from build123d import *

# Parameters (mm, degrees)
F0_W     = 45.72
F0_H     = 3.47472
F1_DEPTH = 3.47472
F3_DEPTH = 3.47472
F5_DEPTH = 38.1
F6_W     = 45.72
F6_H     = 0.254
F7_DEPTH = 0.508
F8_R     = 0.50799


# Not quite as in the source:
# - a fillet or chamfer is up to 0.001 mm smaller than in the source, because OpenCascade refuses the exact size


with BuildPart() as f1:
    # F0 (on Front) → F1 (new body)
    with BuildSketch(Plane.XZ):
        with Locations((0, -4.3103059118)):
            Rectangle(F0_W, F0_H)
    extrude(amount=F1_DEPTH)

    # F2 (on face) → F3 (join)
    with BuildSketch(Plane.XZ.offset(3.47472)):
        Polygon((-13.929602997, -2.5729459118), (-17.4304175377, -2.5729459118), (-24.6292689013, -61.2028853004), (-21.1804489373, -61.6263471453), align=None)
        Polygon((21.1804489373, -61.6263471453), (24.6292689013, -61.2028853004), (17.4304175377, -2.5729459118), (13.929602997, -2.5729459118), align=None)
    extrude(amount=-F3_DEPTH)

    # F4 (on Right) → F5 (cut, symmetric)
    with BuildSketch(Plane.YZ):
        Polygon((-3.47472, -2.9995878813), (0, -2.5729459118), (-3.47472, -2.5729459118), align=None)
        Polygon((0, -60.7762433309), (-3.47472, -61.2028853004), (-3.47472, -61.962287873), (0, -61.962287873), align=None)
    extrude(amount=F5_DEPTH, both=True, mode=Mode.SUBTRACT)

    # F6 (on face) → F7 (cut)
    with BuildSketch(Plane.XZ.offset(3.47472)):
        with Locations((0, -6.1746659118)):
            Rectangle(F6_W, F6_H)
    extrude(amount=-F7_DEPTH, mode=Mode.SUBTRACT)

    # F8 (radius 0.508 in the source; OpenCascade refuses exactly that, so slightly less here)
    f8_edges = [f1.edges().sort_by_distance(p)[0] for p in [
        (0, -3.47472, -2.999588),
        (22.86, 0, -4.310306),
        (22.86, -1.73736, -6.047666),
        (22.86, -3.47472, -4.523627),
        (22.86, -1.73736, -2.786267),
        (21.258758, -3.47472, -33.752276),
        (-17.757943, -3.47472, -33.752276),
        (-21.258758, -3.47472, -33.752276),
        (-22.86, 0, -4.310306),
        (-22.86, -1.73736, -2.786267),
        (-22.86, -3.47472, -4.523627),
        (-22.86, -1.73736, -6.047666),
        (17.757943, -3.47472, -33.752276),
        (20.35853, 0, -6.047666),
        (17.716157, 0, -33.411955),
        (0, 0, -6.047666),
        (-20.35853, 0, -6.047666),
        (-21.216972, 0, -33.411955),
        (-17.716157, 0, -33.411955),
        (21.216972, 0, -33.411955),
        (0, -3.47472, -6.047666),
        (0, 0, -2.572946),
    ]]
    fillet(f8_edges, radius=F8_R)


solid = f1.part
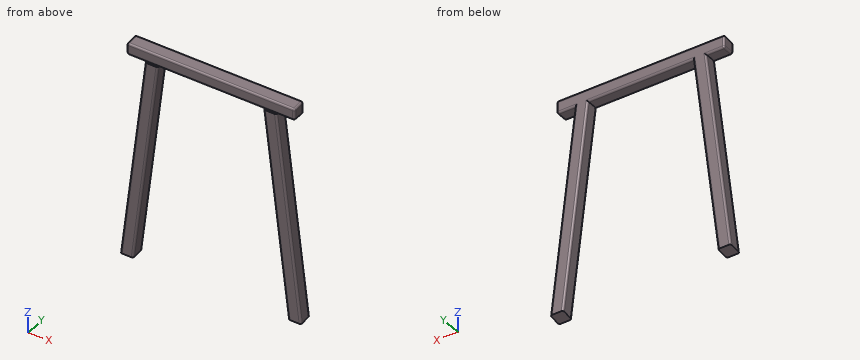
Design review of the part built by this model. Coordinates are the model's own, in mm. Give positions to 0.01 mm unless a question says otherwise; leave off trailing zeros. Loops run counter-clockwise (first coordinate to the right, second up) from the corner with the lowest first, then second, coordinate; pieces in that order, holes last. Notation, with made-up numbers: (86.25, -35) -> (116.25, -35) arc R12 ccw to (116.25, -20) -> close; hole circle Ø5 at (-17, 12.5). An arc over 180 degrees is marked (long way). One line per question, with ' | ' between items. Start each with the question number.
(1) Insertion check: P1, Ø0.7, axis at y = -1.5, z = -4, coming from the +X side; P2, Ø2, axis at x = -9.5, y = -1.5, coming from the -Z side; P3, Ø1.2, axis at y = -1.5, z = -4, coming from the -X side. Each pin has a flat end and moves straight along its axis. Give the tip position at first contact, or say it passes through.
(2) For line 1 (X direction, y = -3, z = -58); line 2 (X direction, y = -0.9, z = -12); line 3 (Z direction, x = -4, y = -0.7), list the stretches that pass through material, from the lowest coordinate up.
(3) We need section A-A (x = 1). State the section outline as (y, z) points.
The answers:
1) P1: stops at x = 22.86 | P2: stops at z = -6.05 | P3: stops at x = -22.86
2) line 1: x = -24.23 to -20.74, 20.74 to 24.23 | line 2: x = -18.59 to -15.09, 15.09 to 18.59 | line 3: z = -6.05 to -2.66
3) outline: (-3.47, -5.54) arc R0.51 ccw to (-2.97, -6.05) -> (-0.51, -6.05) arc R0.51 ccw to (0, -5.54) -> (0, -3.15) arc R0.51 ccw to (-0.57, -2.64) -> (-3.03, -2.94) arc R0.51 ccw to (-3.47, -3.45) -> close
